from build123d import *

# Parameters (mm, degrees)
SKETCH_1_W      = 20
SKETCH_1_H      = 70
EXTRUDE_1_DEPTH = 6
SKETCH_2_W      = 6
SKETCH_2_H      = 70
EXTRUDE_2_DEPTH = 100
EXTRUDE_3_DEPTH = 5


with BuildPart() as part:
    # 草图1 → 凸台-拉伸1 (new body)
    with BuildSketch(Plane(origin=(0, 0, 0), x_dir=(0, 0, -1), z_dir=(1, 0, 0))):
        with Locations((-10, 0)):
            Rectangle(SKETCH_1_W, SKETCH_1_H)
    extrude(amount=EXTRUDE_1_DEPTH)

    # 草图2 → 凸台-拉伸2 (add)
    with BuildSketch(Plane(origin=(6, 0, 0), x_dir=(0, 0, -1), z_dir=(1, 0, 0))):
        with Locations((-3, 0)):
            Rectangle(SKETCH_2_W, SKETCH_2_H)
    extrude(amount=EXTRUDE_2_DEPTH)

    # 草图3 → 凸台-拉伸3 (add)
    with BuildSketch(Plane(origin=(0, 0, 0), x_dir=(-1, 0, 0), z_dir=(0, 0, -1))):
        Polygon((0, -35), (-27.5, -35), (-27.5, -15), (-106, -15), (-106, 15), (-27.5, 15), (-27.5, 35), (0, 35), align=None)
    extrude(amount=EXTRUDE_3_DEPTH)


solid = part.part
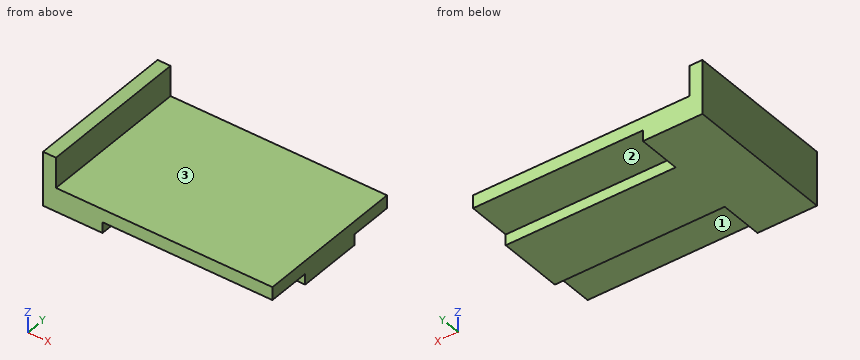
For this review, take the finished solid that the model builds, in its own axes (mm). Face numbers are marked on the shaded views. A direction names the side the tool comes from. Give positions to 0.01 mm unless a question says otherwise; leave off trailing zeros. Loops run counter-clockwise (first coordinate to the right, second up) from the corner with the lowest first, then second, coordinate; pieces in that order, holes last. Notation, with made-up numbers: M 5,-23 L 22,-23 A31 cw 22,12 Z; hole C -13.5,-36 d9. An arc over 180 degrees is marked long. Put each result on its own line as item: value. Start each with the question number.
(1) Machinability: for the marked faces 1, 2 and 3, which of the approach directions +Z, -Z, +X, -X, +Y, -Y give a long, thin tool a straight path to every point of the face, cutting with its end or side? Answer none if there is none.
(2) Add section D-D, the plane z = 11.75. Write out the cut boundary in (x, y), then the cut area to 3 significant figures.
(3) Add section C-C, the plane y = -11. Write out the cut boundary in (x, z), then the cut area to 3 significant figures.
(4) Add section B-B, the plane z = -1.25. Write out the cut boundary in (x, y).
(5) Wall thickness on L1, parallel to Z at x = 46, y = 31.5; L2, parallel to Y at x = 45, z = -2.5: over which ranges is each line inside the solid? List them lowest first.
(6) For pin 1 (6 mm diameter, centred on x = 61, y = 27, fed in from -Z); pin 2 (5 mm diameter, centred on x = 77.5, y = 3.5, fed in from +Z); pin 3 (2.5 mm diameter, centred on x = 64, z = -2.5, fed in from +Y); pin 4 (5 mm diameter, centred on x = 64.5, z = 10, fed in from +Y), all flat-tipped, find the tip position at first contact; note any pin that passes through.
(7) Add section A-A, the plane x = 93. Write out the cut boundary in (y, z), then the cut area to 3 significant figures.
Result:
1. face 1: -Z, +X, -Y
1. face 2: -Z, +X, +Y
1. face 3: +Z, +X, +Y, -Y
2. outline: M 0,-35 L 6,-35 L 6,35 L 0,35 Z
2. area: 420 mm^2
3. outline: M 0,-5 L 106,-5 L 106,6 L 6,6 L 6,20 L 0,20 Z
3. area: 1,250 mm^2
4. outline: M 0,-35 L 27.5,-35 L 27.5,-15 L 106,-15 L 106,15 L 27.5,15 L 27.5,35 L 0,35 Z
5. L1: z = 0 to 6
5. L2: y = -15 to 15
6. pin 1: stops at z = 0
6. pin 2: stops at z = 6
6. pin 3: stops at y = 15
6. pin 4: passes through
7. outline: M -35,0 L -15,0 L -15,-5 L 15,-5 L 15,0 L 35,0 L 35,6 L -35,6 Z
7. area: 570 mm^2
